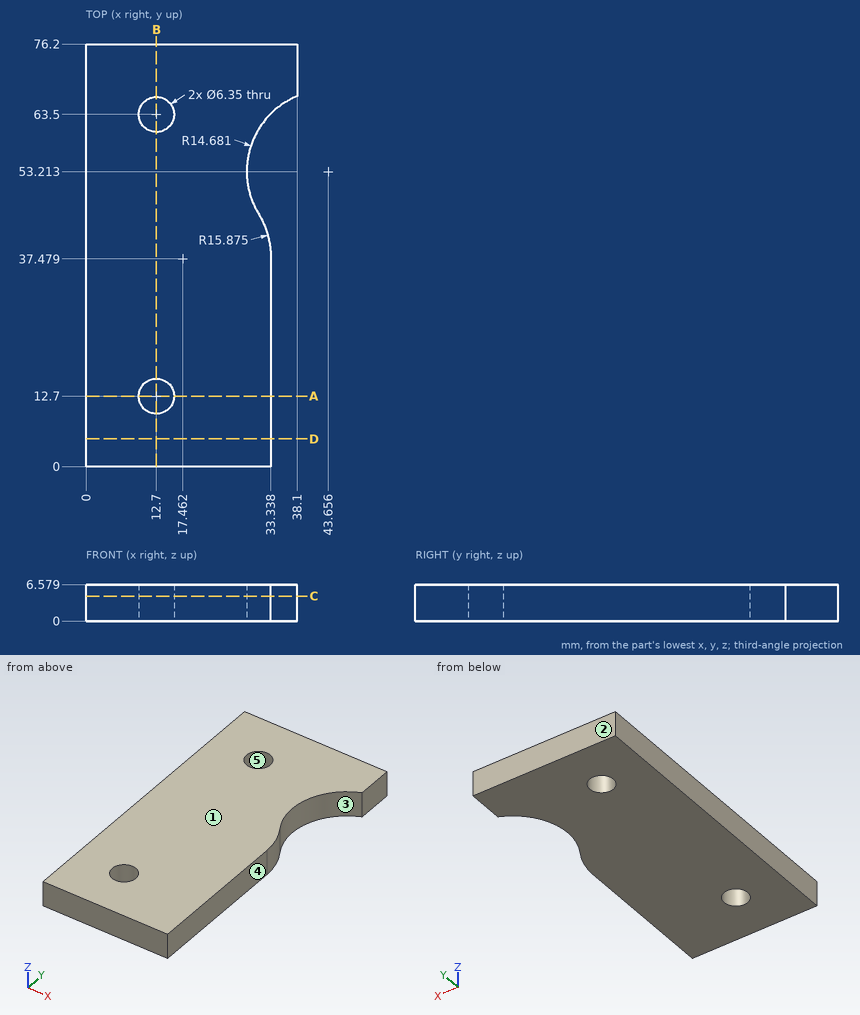
Design review of the part shown in the three views and the two pictorial views. Dimensions are in mm from the part's minimum x, y and z. A direction names the side the tool comes from. Give positions to 0.01 mm unless a question says otherwise; leave off trailing zeros. Loops run counter-clockwise (first coordinate to the right, second up) from the corner with the lowest first, then second, coordinate; pieces in that order, holes last. Notation, with made-up numbers: M -15,-37.75 L 16,-37.75 A5 ccw 16,-33.75 Z; hole C 62,37 d9. An arc over 180 degrees is marked long. Write item = value, one per line.
Q1. We need section C-C (z = 4.5). Count the separate pieces of the cut face and the enclosed holes in it, plus the area to 3 significant figures.
Output values:
separate_pieces = 1
enclosed_holes = 2
area = 2,460 mm^2
Q2. We need section A-A (y = 12.7). Give the boundary of the cut face in (x, z) (1 decimal).
Output values:
outline = M 0,0 L 9.5,0 L 9.5,6.6 L 0,6.6 Z; M 15.9,0 L 33.3,0 L 33.3,6.6 L 15.9,6.6 Z
Q3. To check wall thickness, follow line 1 (Y direction, x = 12.7, z = 1.75) (1 decimal); line 2 (Y direction, x = 14.5, z = 2) (1 decimal); line 3 (X direction, y = 26, z = 0.75). State the ranges of each line that lie inside material, in increasing order. Write a range as [from, to].
Output values:
line_1 = [0, 9.5], [15.9, 60.3], [66.7, 76.2]
line_2 = [0, 10.1], [15.3, 60.9], [66.1, 76.2]
line_3 = [0, 33.34]
Q4. For the marked faces 4 and 5, list the 3-axis set-ups (+Z, -Z, +X, -X, +Y, -Y) from which the entire face can be reached by the end or side of a thin tool; tool diameter is ignored.
Output values:
face_4 = +Z, -Z, +X, -Y
face_5 = +Z, -Z
Q5. Draft analysis for pull direction Y (two halves, no side actions). For the marked faces 1, 2 and 3, state which applies: +Y half, -Y half, draft (parallel to the pull), parting line (faces both ways), or undercut.
Output values:
face_1 = draft
face_2 = +Y half
face_3 = undercut
Q6. Insertion check: pin 1 (3.5 mm diameter, centred on y = 20, z = 2, fed in from +X). The pin has a flat end and moves straight along its axis. Give the tip position at first contact, or say it passes through.
Output values:
pin_1 = 33.34
Q7. We need section B-B (x = 12.7). Give the boundary of the cut face in (y, z) (1 decimal), plus the area to 3 significant figures.
Output values:
outline = M 0,0 L 9.5,0 L 9.5,6.6 L 0,6.6 Z; M 15.9,0 L 60.3,0 L 60.3,6.6 L 15.9,6.6 Z; M 66.7,0 L 76.2,0 L 76.2,6.6 L 66.7,6.6 Z
area = 418 mm^2
Q8. We need section D-D (y = 5). Give the boundary of the cut face in (x, z).
Output values:
outline = M 0,0 L 33.34,0 L 33.34,6.58 L 0,6.58 Z
